```python
from build123d import *

# Parameters (mm, degrees)
SKETCH1_W           = 9
SKETCH1_H           = 23
BOSS_EXTRUDE1_DEPTH = 15
SKETCH2_W           = 7.75
SKETCH2_H           = 3.5
CUT_EXTRUDE1_DEPTH  = 15


with BuildPart() as part:
    # Sketch1 → Boss-Extrude1 (new body)
    with BuildSketch(Plane(origin=(0, 0, 0), x_dir=(1, 0, 0), z_dir=(0, 1, 0))):
        with Locations((4.5, 11.721182832)):
            Rectangle(SKETCH1_W, SKETCH1_H)
    extrude(amount=BOSS_EXTRUDE1_DEPTH)

    # Sketch2 → Cut-Extrude1 (cut)
    with BuildSketch(Plane(origin=(9, 0, 0), x_dir=(0, 0, -1), z_dir=(1, 0, 0))):
        Polygon((0.221182832, 3), (4.83959223, 3), (4.83959223, 6.5), (18.58959223, 6.5), (18.58959223, 3), (23.221182832, 3), (23.221182832, 15), (0.221182832, 15), align=None)
        with Locations((11.71459223, 1.75)):
            Rectangle(SKETCH2_W, SKETCH2_H)
    extrude(amount=-CUT_EXTRUDE1_DEPTH, mode=Mode.SUBTRACT)


solid = part.part
```
Part model, mm, in its own coordinate system. A direction names the side the tool comes from. Give positions to 0.01 mm unless a question says otherwise; leave off trailing zeros. Loops run counter-clockwise (first coordinate to the right, second up) from the corner with the lowest first, then second, coordinate; pieces in that order, holes last. Notation, with made-up numbers: M 16,87 L 55,87 A22 ccw 55,111 Z; hole C 64,33 d1. An arc over 180 degrees is marked long. Return JSON: item names as keys, results as strings.
1) 3-axis set-ups, long thin cutter, end or side, ignore diameter. For faces 4 (the face through (5, 5, -4.84)), 5 (the face through (5, 5, -18.59)), 6 (the face through (5, 2, -7.84)): which of +Z, -Z, +X, -X, +Y, -Y reach the whole face in a straight line?
Calculated:
{"face 4": "+Z, +X, -X, +Y", "face 5": "-Z, +X, -X, +Y", "face 6": "+X, -X, -Y"}
2) Pull direction Z, two halves, no side cores. Call faces 1 (the face through (4, 1, -0.221)), 2 (the face through (5, 3, -2)), 3 (the face through (5, 2, -15.59)): released by +Z, released by -Z, zero draft, split by the parting line, or undercut.
Calculated:
{"face 1": "released by +Z", "face 2": "zero draft", "face 3": "undercut"}
3) Saw through at A-A, the plane y = 2.5. List the corners of the cut face in (x, z), then the cut area to 3 significant figures.
Calculated:
{"outline": "M 0,-23.22 L 9,-23.22 L 9,-15.59 L 0,-15.59 Z; M 0,-7.84 L 9,-7.84 L 9,-0.22 L 0,-0.22 Z", "area": "137 mm2"}
4) Flat gauge pins, fed straight in: pin 1 Ø3.5 at (x, z) = (5, -2.5) entering from +Y; pin 2 Ø4 at (x, z) = (5, -12.5) entering from -Y. Where does each tip first touch, or does it go through?
Calculated:
{"pin 1": "stops at y = 3", "pin 2": "stops at y = 3.5"}
5) Drill centre lines: line 1 (Z direction, x = 7.25, y = 0.75); line 2 (Z direction, x = 3.5, y = 4.25); line 3 (Y direction, x = 6.25, z = -14.5). Where is each one in solid material? Low to high.
Calculated:
{"line 1": "z = -23.22 to -15.59, -7.84 to -0.22", "line 2": "z = -18.59 to -4.84", "line 3": "y = 3.5 to 6.5"}
6) Saw through at C-C, the plane z = -13.75. List the corners of the cut face in (x, y).
Calculated:
{"outline": "M 0,3.5 L 9,3.5 L 9,6.5 L 0,6.5 Z"}
7) Saw through at B-B, the plane x = 5.5. List the corners of the cut face in (y, z), then the cut area to 3 significant figures.
Calculated:
{"outline": "M 0,-23.22 L 3,-23.22 L 3,-18.59 L 6.5,-18.59 L 6.5,-4.84 L 3,-4.84 L 3,-0.22 L 0,-0.22 L 0,-7.84 L 3.5,-7.84 L 3.5,-15.59 L 0,-15.59 Z", "area": "90.0 mm2"}
